Check sheet for the modelled part. Datum: model origin and axes. Units: mm. A direction names the side the tool comes from. Give positions to 0.01 mm unless a question says otherwise; leave off trailing zeros. Write each loop counter-clockwise with the first axis right and the second up, starting at its lowest first coordinate (ties: lowest second). Pieces come first, ordered by that corner, then holes. Notation, with made-up numbers: (-2.5, -33.5) -> (34.5, -33.5) arc R20 ccw to (34.5, -12.5) -> close; hole circle Ø1 at (78.25, 51.5). An arc over 180 degrees is marked (long way). Use a Markdown table: item, result. Add a question column.
1. Release check for a two-part mould opening along X. For faces 1 (the flat face through (-21.726, -2, 19)), 2 (the flat face through (11.274, -2, -31)), 3 (the flat face through (44.274, -2, -16)), 4 (the flat face through (7, -3, -6)) record: released by +X, released by -X, zero draft, split by the parting line, or undercut.
2. Cross-section at A-A (y = -0.85). Enter the section's corners in (x, z).
3. Cross-section at B-B (z = -6). Enter the section's corners in (x, y).
4. Scan lines: probe 1 along X at (y, z) = (-0.9, 1); probe 2 along Z at (x, y) = (45.5, -1.35); probe 3 along Z at (x, y) = (12, -1.6). Record each from-to range of solid material in increasing order. Write a range as [from, to].
5. Gauge pin test, flat ends, axial feed: P1, Ø0.9, axis at x = -22.5, y = -1, coming from the +Z side; P2, Ø1.5, axis at x = 13, y = -2, coming from the -Z side; P3, Ø1.5, axis at y = -1, z = 18.5, coming from the -X side. Record the tip position at first contact, or that the pin passes through.
6. Set-up check for faces 5 (the flat face through (44.274, -2, 19)), 6 (the flat face through (59.274, -1, 10)), 7 (the flat face through (52, -2, 1.126)), 8 (the flat face through (14.274, -2, -31)), 9 (the flat face through (-23, -2, 17.126)): record each of +Z, -Z, +X, -X, +Y, -Y from which the full face is reachable in a straight line by a thin tool's end or side.
from build123d import *

# Parameters (mm, degrees)
F0_W     = 84
F0_H     = 53
F1_DEPTH = 3
F2_W     = 15
F2_H     = 34
F3_DEPTH = 25
F4_W     = 4
F4_H     = 3
F5_DEPTH = 25
F6_W     = 3
F6_H     = 3
F7_DEPTH = 25
F8_W     = 3
F8_H     = 3
F9_DEPTH = 25


with BuildPart() as f1:
    # F0 (on Front) → F1 (new body)
    with BuildSketch(Plane.XZ):
        with Locations((17.273909, -6.373649)):
            Rectangle(F0_W, F0_H)
    extrude(amount=F1_DEPTH)

    # F2 (on face) → F3 (cut)
    with BuildSketch(Plane.XZ.offset(3)):
        with Locations((51.773909, -15.873649)):
            Rectangle(F2_W, F2_H)
    extrude(amount=-F3_DEPTH, mode=Mode.SUBTRACT)

    # F4 (on face) → F5 (cut)
    with BuildSketch(Plane.XZ.offset(3)):
        with Locations((42.273909, 18.626351)):
            Rectangle(F4_W, F4_H)
    extrude(amount=-F5_DEPTH, mode=Mode.SUBTRACT)

    # F6 (on face) → F7 (cut)
    with BuildSketch(Plane.XZ.offset(3)):
        with Locations((-23.226091, 18.626351)):
            Rectangle(F6_W, F6_H)
    extrude(amount=-F7_DEPTH, mode=Mode.SUBTRACT)

    # F8 (on face) → F9 (cut)
    with BuildSketch(Plane.XZ.offset(3)):
        with Locations((12.773909, -31.373649)):
            Rectangle(F8_W, F8_H)
    extrude(amount=-F9_DEPTH, mode=Mode.SUBTRACT)


solid = f1.part
Worked answers:
| question | item | result |
|---|---|---|
| 1 | face 1 | released by -X |
| 1 | face 2 | undercut |
| 1 | face 3 | released by +X |
| 1 | face 4 | zero draft |
| 2 | outline | (-24.73, -32.87) -> (11.27, -32.87) -> (11.27, -29.87) -> (14.27, -29.87) -> (14.27, -32.87) -> (44.27, -32.87) -> (44.27, 1.13) -> (59.27, 1.13) -> (59.27, 20.13) -> (44.27, 20.13) -> (44.27, 17.13) -> (40.27, 17.13) -> (40.27, 20.13) -> (-21.73, 20.13) -> (-21.73, 17.13) -> (-24.73, 17.13) -> close |
| 3 | outline | (-24.73, -3) -> (44.27, -3) -> (44.27, 0) -> (-24.73, 0) -> close |
| 4 | probe 1 | x = [-24.73, 44.27] |
| 4 | probe 2 | z = [1.13, 20.13] |
| 4 | probe 3 | z = [-29.87, 20.13] |
| 5 | P1 | stops at z = 17.13 |
| 5 | P2 | stops at z = -29.87 |
| 5 | P3 | stops at x = -21.73 |
| 6 | face 5 | +Z, +Y, -Y |
| 6 | face 6 | +Z, -Z, +X, +Y, -Y |
| 6 | face 7 | -Z, +X, +Y, -Y |
| 6 | face 8 | -Z, +Y, -Y |
| 6 | face 9 | +Z, -X, +Y, -Y |
